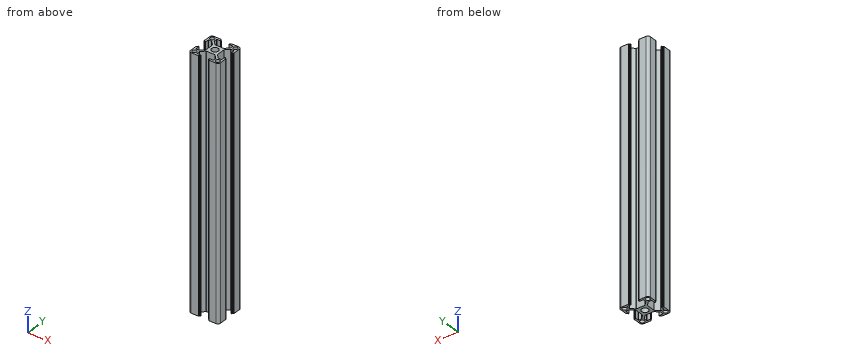
from build123d import *

# Parameters (mm, degrees)
CROQUIS1_R              = 2.1
CROQUIS1_R_2            = 3.4
SALIENTE_EXTRUIR1_DEPTH = 400
CROQUIS3_W              = 36.891585518
CROQUIS3_H              = 31.857253434
CORTAR_EXTRUIR2_DEPTH   = 150


with BuildPart() as part:
    # Croquis1 → Saliente-Extruir1 (new body)
    with BuildSketch(Plane(origin=(0, 0, -50), x_dir=(-1, 0, 0), z_dir=(0, 0, -1))):
        with BuildLine():
            Line((14.7, -5.1), (14.3, -5.1))
            ThreePointArc((14.3, -5.1), (14.087867966, -5.012132034), (14, -4.8))
            Line((14, -4.8), (14, -4.4))
            ThreePointArc((14, -4.4), (13.912132034, -4.187867966), (13.7, -4.1))
            Line((13.7, -4.1), (13.3, -4.1))
            ThreePointArc((13.3, -4.1), (13.087867966, -4.187867966), (13, -4.4))
            Line((13, -4.4), (13, -7.95))
            ThreePointArc((13, -7.95), (12.912132034, -8.162132034), (12.7, -8.25))
            Line((12.7, -8.25), (9.789264108, -8.25))
            ThreePointArc((9.789264108, -8.25), (9.674477865, -8.22717164), (9.577160832, -8.162160788))
            Line((9.577160832, -8.162160788), (5.887896723, -4.473896751))
            ThreePointArc((5.887896723, -4.473896751), (5.822843922, -4.376559778), (5.8, -4.261735963))
            Line((5.8, -4.261735963), (5.8, 4.260735931))
            ThreePointArc((5.8, 4.260735931), (5.82283614, 4.375540961), (5.887867966, 4.472867966))
            Line((5.887867966, 4.472867966), (9.577132034, 8.162132034))
            ThreePointArc((9.577132034, 8.162132034), (9.674459039, 8.22716386), (9.789264069, 8.25))
            Line((9.789264069, 8.25), (12.7, 8.25))
            ThreePointArc((12.7, 8.25), (12.912132034, 8.162132034), (13, 7.95))
            Line((13, 7.95), (13, 4.4))
            ThreePointArc((13, 4.4), (13.087867966, 4.187867966), (13.3, 4.1))
            Line((13.3, 4.1), (13.7, 4.1))
            ThreePointArc((13.7, 4.1), (13.912132034, 4.187867966), (14, 4.4))
            Line((14, 4.4), (14, 4.8))
            ThreePointArc((14, 4.8), (14.087867966, 5.012132034), (14.3, 5.1))
            Line((14.3, 5.1), (14.7, 5.1))
            ThreePointArc((14.7, 5.1), (14.912132034, 5.187867966), (15, 5.4))
            Line((15, 5.4), (15, 12.5))
            ThreePointArc((15, 12.5), (14.267766953, 14.267766953), (12.5, 15))
            Line((12.5, 15), (5.4, 15))
            ThreePointArc((5.4, 15), (5.187867966, 14.912132034), (5.1, 14.7))
            Line((5.1, 14.7), (5.1, 14.3))
            ThreePointArc((5.1, 14.3), (5.012132034, 14.087867966), (4.8, 14))
            Line((4.8, 14), (4.4, 14))
            ThreePointArc((4.4, 14), (4.187867966, 13.912132034), (4.1, 13.7))
            Line((4.1, 13.7), (4.1, 13.3))
            ThreePointArc((4.1, 13.3), (4.187867966, 13.087867966), (4.4, 13))
            Line((4.4, 13), (7.95, 13))
            ThreePointArc((7.95, 13), (8.162132034, 12.912132034), (8.25, 12.7))
            Line((8.25, 12.7), (8.25, 9.788264069))
            ThreePointArc((8.25, 9.788264069), (8.22716386, 9.673459039), (8.162132034, 9.576132034))
            Line((8.162132034, 9.576132034), (4.473867966, 5.887867966))
            ThreePointArc((4.473867966, 5.887867966), (4.376540961, 5.82283614), (4.261735931, 5.8))
            Line((4.261735931, 5.8), (-4.260735892, 5.8))
            ThreePointArc((-4.260735892, 5.8), (-4.375522135, 5.82282836), (-4.472839168, 5.887839212))
            Line((-4.472839168, 5.887839212), (-8.162103277, 9.576103249))
            ThreePointArc((-8.162103277, 9.576103249), (-8.227156078, 9.673440222), (-8.25, 9.788264037))
            Line((-8.25, 9.788264037), (-8.25, 12.7))
            ThreePointArc((-8.25, 12.7), (-8.162132034, 12.912132034), (-7.95, 13))
            Line((-7.95, 13), (-4.4, 13))
            ThreePointArc((-4.4, 13), (-4.187867966, 13.087867966), (-4.1, 13.3))
            Line((-4.1, 13.3), (-4.1, 13.7))
            ThreePointArc((-4.1, 13.7), (-4.187867966, 13.912132034), (-4.4, 14))
            Line((-4.4, 14), (-4.8, 14))
            ThreePointArc((-4.8, 14), (-5.012132034, 14.087867966), (-5.1, 14.3))
            Line((-5.1, 14.3), (-5.1, 14.7))
            ThreePointArc((-5.1, 14.7), (-5.187867966, 14.912132034), (-5.4, 15))
            Line((-5.4, 15), (-12.5, 15))
            ThreePointArc((-12.5, 15), (-14.267766953, 14.267766953), (-15, 12.5))
            Line((-15, 12.5), (-15, 5.4))
            ThreePointArc((-15, 5.4), (-14.912132034, 5.187867966), (-14.7, 5.1))
            Line((-14.7, 5.1), (-14.3, 5.1))
            ThreePointArc((-14.3, 5.1), (-14.087867966, 5.012132034), (-14, 4.8))
            Line((-14, 4.8), (-14, 4.4))
            ThreePointArc((-14, 4.4), (-13.912132034, 4.187867966), (-13.7, 4.1))
            Line((-13.7, 4.1), (-13.3, 4.1))
            ThreePointArc((-13.3, 4.1), (-13.087867966, 4.187867966), (-13, 4.4))
            Line((-13, 4.4), (-13, 7.95))
            ThreePointArc((-13, 7.95), (-12.912132034, 8.162132034), (-12.7, 8.25))
            Line((-12.7, 8.25), (-9.788264037, 8.25))
            ThreePointArc((-9.788264037, 8.25), (-9.673440222, 8.227156078), (-9.576103249, 8.162103277))
            Line((-9.576103249, 8.162103277), (-5.887839212, 4.472839168))
            ThreePointArc((-5.887839212, 4.472839168), (-5.82282836, 4.375522135), (-5.8, 4.260735892))
            Line((-5.8, 4.260735892), (-5.8, -4.261735931))
            ThreePointArc((-5.8, -4.261735931), (-5.82283614, -4.376540961), (-5.887867966, -4.473867966))
            Line((-5.887867966, -4.473867966), (-9.576132034, -8.162132034))
            ThreePointArc((-9.576132034, -8.162132034), (-9.673459039, -8.22716386), (-9.788264069, -8.25))
            Line((-9.788264069, -8.25), (-12.7, -8.25))
            ThreePointArc((-12.7, -8.25), (-12.912132034, -8.162132034), (-13, -7.95))
            Line((-13, -7.95), (-13, -4.4))
            ThreePointArc((-13, -4.4), (-13.087867966, -4.187867966), (-13.3, -4.1))
            Line((-13.3, -4.1), (-13.7, -4.1))
            ThreePointArc((-13.7, -4.1), (-13.912132034, -4.187867966), (-14, -4.4))
            Line((-14, -4.4), (-14, -4.8))
            ThreePointArc((-14, -4.8), (-14.087867966, -5.012132034), (-14.3, -5.1))
            Line((-14.3, -5.1), (-14.7, -5.1))
            ThreePointArc((-14.7, -5.1), (-14.912132034, -5.187867966), (-15, -5.4))
            Line((-15, -5.4), (-15, -12.5))
            ThreePointArc((-15, -12.5), (-14.267766953, -14.267766953), (-12.5, -15))
            Line((-12.5, -15), (-5.4, -15))
            ThreePointArc((-5.4, -15), (-5.187867966, -14.912132034), (-5.1, -14.7))
            Line((-5.1, -14.7), (-5.1, -14.3))
            ThreePointArc((-5.1, -14.3), (-5.012132034, -14.087867966), (-4.8, -14))
            Line((-4.8, -14), (-4.4, -14))
            ThreePointArc((-4.4, -14), (-4.187867966, -13.912132034), (-4.1, -13.7))
            Line((-4.1, -13.7), (-4.1, -13.3))
            ThreePointArc((-4.1, -13.3), (-4.187867966, -13.087867966), (-4.4, -13))
            Line((-4.4, -13), (-7.95, -13))
            ThreePointArc((-7.95, -13), (-8.162132034, -12.912132034), (-8.25, -12.7))
            Line((-8.25, -12.7), (-8.25, -9.789264069))
            ThreePointArc((-8.25, -9.789264069), (-8.22716386, -9.674459039), (-8.162132034, -9.577132034))
            Line((-8.162132034, -9.577132034), (-4.472867966, -5.887867966))
            ThreePointArc((-4.472867966, -5.887867966), (-4.375540961, -5.82283614), (-4.260735931, -5.8))
            Line((-4.260735931, -5.8), (4.261735963, -5.8))
            ThreePointArc((4.261735963, -5.8), (4.376559778, -5.822843922), (4.473896751, -5.887896723))
            Line((4.473896751, -5.887896723), (8.162160788, -9.577160832))
            ThreePointArc((8.162160788, -9.577160832), (8.22717164, -9.674477865), (8.25, -9.789264108))
            Line((8.25, -9.789264108), (8.25, -12.7))
            ThreePointArc((8.25, -12.7), (8.162132034, -12.912132034), (7.95, -13))
            Line((7.95, -13), (4.4, -13))
            ThreePointArc((4.4, -13), (4.187867966, -13.087867966), (4.1, -13.3))
            Line((4.1, -13.3), (4.1, -13.7))
            ThreePointArc((4.1, -13.7), (4.187867966, -13.912132034), (4.4, -14))
            Line((4.4, -14), (4.8, -14))
            ThreePointArc((4.8, -14), (5.012132034, -14.087867966), (5.1, -14.3))
            Line((5.1, -14.3), (5.1, -14.7))
            ThreePointArc((5.1, -14.7), (5.187867966, -14.912132034), (5.4, -15))
            Line((5.4, -15), (12.5, -15))
            ThreePointArc((12.5, -15), (14.267766953, -14.267766953), (15, -12.5))
            Line((15, -12.5), (15, -5.4))
            ThreePointArc((15, -5.4), (14.912132034, -5.187867966), (14.7, -5.1))
        make_face()
        with Locations((-11.7, 11.7)):
            Circle(CROQUIS1_R, mode=Mode.SUBTRACT)
        with Locations((-11.7, -11.7)):
            Circle(CROQUIS1_R, mode=Mode.SUBTRACT)
        Circle(CROQUIS1_R_2, mode=Mode.SUBTRACT)
        with Locations((11.7, 11.7)):
            Circle(CROQUIS1_R, mode=Mode.SUBTRACT)
        with Locations((11.7, -11.7)):
            Circle(CROQUIS1_R, mode=Mode.SUBTRACT)
    extrude(amount=-SALIENTE_EXTRUIR1_DEPTH)

    # Croquis3 → Cortar-Extruir2 (cut)
    with BuildSketch(Plane(origin=(0, 0, -50), x_dir=(-1, 0, 0), z_dir=(0, 0, -1))):
        with Locations((0.583982522, 0.302059925)):
            Rectangle(CROQUIS3_W, CROQUIS3_H)
    extrude(amount=-CORTAR_EXTRUIR2_DEPTH, mode=Mode.SUBTRACT)


solid = part.part
Input: part model. Units: mm. Frame: model coordinates. Round coordinates to 2 decimals unless told otherwise and drop trailing zeros. Order: outer loops, then holes, each group sorted by start corner. A loop starts at its lowest first (then second) coordinate and runs counter-clockwise, first axis right, second up. Notation, with made-up numbers: (-35, 25.25) - (8, 25.25) arc R23 cw to (8, 42.25) - close; hole circle Ø6 at (12.25, 61.25). An arc over 180 degrees is marked (long way). Answer as a JSON object with one key per item and string values. Group by question number.
(1) Cut plane C-C (z = 244). Count the separate pieces of the cut face and the enclosed holes in it, then the cut area to 3 significant figures.
(2) Cut plane A-A (y = 0). Return loops of the section in (x, z), then the cut area to 3 significant figures.
(3) Material intervals for probe 1 along Y at (x, z) = (-11.7, 209); probe 2 along X at (y, z) = (6, 284.5) (3 decimals); probe 3 along Y at (x, z) = (-7.75, 233.5) (1 decimal), sorted ascending. Write a range as from..to.
(4) Pin query (flat end, axial travel): P1, Ø3, axis at y = -2, z = 259, coming from the +X side; P2, Ø3, axis at x = 0.5, z = 219.5, coming from the +Y side. Return the tip coordinate at first contact, or that it passes through.
Here are the results:
{
 "1": {"separate pieces": "1", "enclosed holes": "5", "area": "314 mm^2"},
 "2": {"outline": "(-5.8, 100) - (-3.4, 100) - (-3.4, 350) - (-5.8, 350) - close; (3.4, 100) - (5.8, 100) - (5.8, 350) - (3.4, 350) - close", "area": "1,200 mm^2"},
 "3": {"probe 1": "y = -15..-13.8, -9.6..-8.25, 8.25..9.6, 13.8..15", "probe 2": "x = -15..-13, -7.415..-4.586, 4.585..7.415, 13..15", "probe 3": "y = -15..-13, -9.2..-6.3, 6.3..9.2, 13..15"},
 "4": {"P1": "stops at x = 5.8", "P2": "stops at y = 5.8"}
}
